from build123d import *

# Parameters (mm, degrees)
SKETCH_1_W          = 15
SKETCH_1_H          = 15
SKETCH_1_W_2        = 13
SKETCH_1_H_2        = 13
EXTRUDE_1_DEPTH     = 215
CUT_EXTRUDE_1_REACH = 218.044
SKETCH_2_R          = 2


with BuildPart() as part:
    # ｽｹｯﾁ1 → 押し出し-薄板1 (new body)
    with BuildSketch(Plane(origin=(0, 0, 0), x_dir=(0, 0, -1), z_dir=(1, 0, 0))):
        with Locations((7.5, 7.5)):
            Rectangle(SKETCH_1_W, SKETCH_1_H)
        with Locations((7.5, 7.5)):
            Rectangle(SKETCH_1_W_2, SKETCH_1_H_2, mode=Mode.SUBTRACT)
    extrude(amount=EXTRUDE_1_DEPTH)

    # ｶｯﾄ - 押し出し1: up to this face of the body (flat: up to its plane)
    cut_extrude_1_end = Plane(part.part.faces().sort_by_distance((107.5, 0, -7.5))[0])
    # ｽｹｯﾁ2 → ｶｯﾄ - 押し出し1 (cut, up to the picked face)
    with BuildSketch(Plane(origin=(0, 15, 0), x_dir=(1, 0, 0), z_dir=(0, 1, 0)), mode=Mode.PRIVATE) as cut_extrude_1_sk1:
        with Locations(Location((107.5, 7.5, 0), (0, 0, 270))):
            Circle(SKETCH_2_R)
    cut_extrude_1_tool1 = split(extrude(cut_extrude_1_sk1.sketch, amount=-CUT_EXTRUDE_1_REACH, mode=Mode.PRIVATE), bisect_by=cut_extrude_1_end, keep=Keep.BOTH, mode=Mode.PRIVATE)
    # ｽｹｯﾁ2 → ｶｯﾄ - 押し出し1 (cut, up to the picked face)
    with BuildSketch(Plane(origin=(0, 15, 0), x_dir=(1, 0, 0), z_dir=(0, 1, 0)), mode=Mode.PRIVATE) as cut_extrude_1_sk2:
        with Locations(Location((7.5, 7.5, 0), (0, 0, 270))):
            Circle(SKETCH_2_R)
    cut_extrude_1_tool2 = split(extrude(cut_extrude_1_sk2.sketch, amount=-CUT_EXTRUDE_1_REACH, mode=Mode.PRIVATE), bisect_by=cut_extrude_1_end, keep=Keep.BOTH, mode=Mode.PRIVATE)
    # ｽｹｯﾁ2 → ｶｯﾄ - 押し出し1 (cut, up to the picked face)
    with BuildSketch(Plane(origin=(0, 15, 0), x_dir=(1, 0, 0), z_dir=(0, 1, 0)), mode=Mode.PRIVATE) as cut_extrude_1_sk3:
        with Locations(Location((207.5, 7.5, 0), (0, 0, 90))):
            Circle(SKETCH_2_R)
    cut_extrude_1_tool3 = split(extrude(cut_extrude_1_sk3.sketch, amount=-CUT_EXTRUDE_1_REACH, mode=Mode.PRIVATE), bisect_by=cut_extrude_1_end, keep=Keep.BOTH, mode=Mode.PRIVATE)
    # ｽｹｯﾁ2 → ｶｯﾄ - 押し出し1 (cut, up to the picked face)
    with BuildSketch(Plane(origin=(0, 15, 0), x_dir=(1, 0, 0), z_dir=(0, 1, 0)), mode=Mode.PRIVATE) as cut_extrude_1_sk4:
        with Locations(Location((148, 7.5, 0), (0, 0, 270))):
            Circle(SKETCH_2_R)
    cut_extrude_1_tool4 = split(extrude(cut_extrude_1_sk4.sketch, amount=-CUT_EXTRUDE_1_REACH, mode=Mode.PRIVATE), bisect_by=cut_extrude_1_end, keep=Keep.BOTH, mode=Mode.PRIVATE)
    add(cut_extrude_1_tool1.solids().sort_by(Axis((107.5, 15, -7.5), (0, -1, 0)))[0], mode=Mode.SUBTRACT)
    add(cut_extrude_1_tool2.solids().sort_by(Axis((7.5, 15, -7.5), (0, -1, 0)))[0], mode=Mode.SUBTRACT)
    add(cut_extrude_1_tool3.solids().sort_by(Axis((207.5, 15, -7.5), (0, -1, 0)))[0], mode=Mode.SUBTRACT)
    add(cut_extrude_1_tool4.solids().sort_by(Axis((148, 15, -7.5), (0, -1, 0)))[0], mode=Mode.SUBTRACT)


solid = part.part
Source: CAD feature listing. Evaluate the final solid. Frame: model axes, mm. A direction names the side the tool comes from. Coordinates: 2 decimals unless noted, no trailing zeros. Loops run counter-clockwise (first coordinate to the right, second up) from the corner with the lowest first, then second, coordinate; pieces in that order, holes last. Notation, with made-up numbers: (62, 23) - (108, 23) arc R30 ccw to (108, 61) - close; hole circle Ø3 at (31.25, 79). An arc over 180 degrees is marked (long way). One line per item, written item: value. Start each with the question number.
1. Set-up query: faces 4 (the flat face through (106, 14, -10)), 5 (the cylindrical face through (109.483, 0.507, -7.76)). Return all of +Z, -Z, +X, -X, +Y, -Y with unobstructed straight access to the full face (end or side cutting, diameter ignored); none if empty.
2. Section A-A (y = 4). Return the cut outline in (x, z), and give its area (3 significant figures).
3. Section C-C (x = 46.5). Return the cut outline in (y, z).
4. Ray query, L1, parallel to X at y = 14.25, z = -7.5; L2, parallel to Y at x = 101, z = -12; L3, parallel to Z at x = 53.5, y = 12.75. Return the intervals inside material, ascending.
5. Mould query, pull axis X, two halves, no side actions, for faces 1 (the flat face through (106, 7, -15)), 2 (the cylindrical face through (146.226, 0.507, -6.577)), 3 (the flat face through (215, 7.6, -0.7)). Classes: pulls with the +X half, pulls with the -X half, needs draft (parallel to the pull), parting line crosses it, or undercut.
6. Section B-B (x = 207.5). Return the cut outline in (y, z).
7. Section D-D (z = -7.5). State how many separate pieces and enclosed holes the cut face has, and give its area (3 significant figures).
Verdict:
1. face 4: +X, -X
1. face 5: +Y, -Y
2. outline: (0, -15) - (215, -15) - (215, -14) - (0, -14) - close; (0, -1) - (215, -1) - (215, 0) - (0, 0) - close
2. area: 430 mm2
3. outline: (0, -15) - (15, -15) - (15, 0) - (0, 0) - close; hole (1, -14) - (14, -14) - (14, -1) - (1, -1) - close
4. L1: x = 0 to 5.5, 9.5 to 105.5, 109.5 to 146, 150 to 205.5, 209.5 to 215
4. L2: y = 0 to 1, 14 to 15
4. L3: z = -15 to -14, -1 to 0
5. face 1: needs draft
5. face 2: undercut
5. face 3: pulls with the +X half
6. outline: (0, -15) - (15, -15) - (15, -9.5) - (14, -9.5) - (14, -14) - (1, -14) - (1, -9.5) - (0, -9.5) - close; (0, -5.5) - (1, -5.5) - (1, -1) - (14, -1) - (14, -5.5) - (15, -5.5) - (15, 0) - (0, 0) - close
7. separate pieces: 10
7. enclosed holes: 0
7. area: 398 mm2
